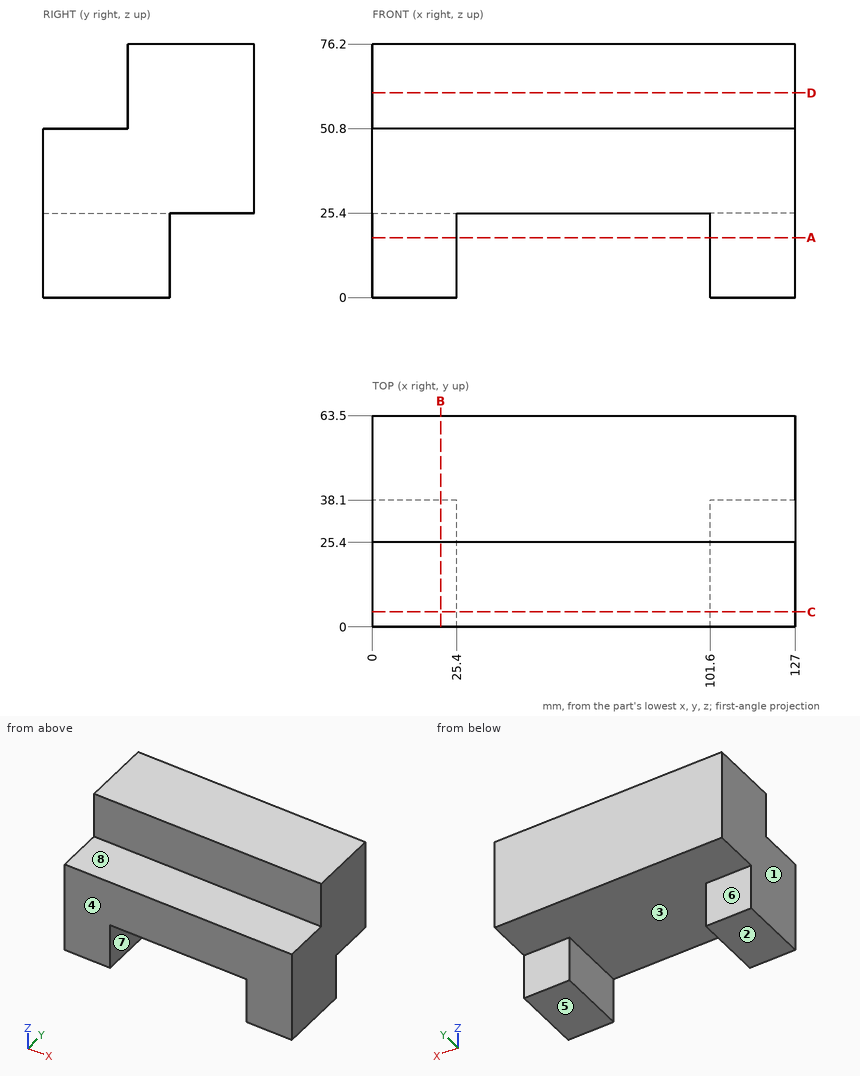
Design review of the part shown in the three views and the two pictorial views. Dimensions are in mm from the part's minimum x, y and z. A direction names the side the tool comes from. Give positions to 0.01 mm unless a question says otherwise; leave off trailing zeros. Loops run counter-clockwise (first coordinate to the right, second up) from the corner with the lowest first, then second, coordinate; pieces in that order, holes last. Notation, with made-up numbers: (-3, 73) -> (11, 73) arc R11 ccw to (11, 77) -> close; hole circle Ø7 at (-39.75, 82). An arc over 180 degrees is marked (long way). Put each result on its own line as item: value. Start each with the question number.
1. Wall thickness on probe 1 along X at (y, z) = (34, 10.5); probe 2 along Z at (x, y) = (26.5, 54); probe 3 along Y at (x, z) = (14.5, 23.5): over which ranges is each line inside the solid? List them lowest first.
2. We need section A-A on z = 18. State the section outline as (x, y) points, then the cut area to 3 significant figures.
3. For the marked faces 4, 5, 6, 7 and 8, list the 3-axis set-ups (+Z, -Z, +X, -X, +Y, -Y) from which the entire face can be reached by the end or side of a thin tool; tool diameter is ignored.
4. We need section B-B on x = 20.5. State the section outline as (y, z) points, then the cut area to 3 significant figures.
5. Mouldability with a two-part tool opening along X and no side actions: class the marked faces 1, 2 and 3 as released by +X, released by -X, zero draft, split by the parting line, or undercut.
6. We need section D-D on z = 61.5. State the section outline as (x, y) points, then the cut area to 3 significant figures.
7. We need section C-C on y = 4.5. State the section outline as (x, z) points, then the cut area to 3 significant figures.
8. Clearance check with flat-ended pins moving along their axes: P1, Ø3, axis at x = 108, z = 64.5, coming from the -Y side; P2, Ø8, axis at x = 63, y = 51.5, coming from the -Z side; P3, Ø6, axis at x = 51, z = 21, coming from the -Y side; P4, Ø20.5, axis at x = 9.5, z = 7.5, coming from the +Y side. State where each tip first meets the part, or that it passes through.
Determined:
1. probe 1: 0 to 25.4, 101.6 to 127
1. probe 2: 25.4 to 76.2
1. probe 3: 0 to 38.1
2. outline: (0, 0) -> (25.4, 0) -> (25.4, 38.1) -> (0, 38.1) -> close; (101.6, 0) -> (127, 0) -> (127, 38.1) -> (101.6, 38.1) -> close
2. area: 1,940 mm^2
3. face 4: +Z, -Z, +X, -X, -Y
3. face 5: -Z, +X, -X, +Y, -Y
3. face 6: -Z, +X, -X, +Y
3. face 7: -Z, +Y, -Y
3. face 8: +Z, +X, -X, -Y
4. outline: (0, 0) -> (38.1, 0) -> (38.1, 25.4) -> (63.5, 25.4) -> (63.5, 76.2) -> (25.4, 76.2) -> (25.4, 50.8) -> (0, 50.8) -> close
4. area: 3,550 mm^2
5. face 1: released by -X
5. face 2: zero draft
5. face 3: undercut
6. outline: (0, 25.4) -> (127, 25.4) -> (127, 63.5) -> (0, 63.5) -> close
6. area: 4,840 mm^2
7. outline: (0, 0) -> (25.4, 0) -> (25.4, 25.4) -> (101.6, 25.4) -> (101.6, 0) -> (127, 0) -> (127, 50.8) -> (0, 50.8) -> close
7. area: 4,520 mm^2
8. P1: y = 25.4
8. P2: z = 25.4
8. P3: through
8. P4: y = 38.1
